from build123d import *

# Parameters (mm, degrees)
REFERENCE_R         = 6.35
REFERENCE_R_2       = 3.175
REFERENCE_R_3       = 2.0955
REFERENCE_R_4       = 1.9685
REFERENCE_R_5       = 2.032
BOSS_EXTRUDE3_DEPTH = 6.604


with BuildPart() as part:
    # reference → Boss-Extrude3 (new body)
    with BuildSketch(Plane.XY):
        Polygon((209.55, 0), (-209.55, 0), (-209.55, 170.18), (-74.93, 304.8), (74.93, 304.8), (209.55, 170.18), align=None)
        with Locations(Location((-102.87, 111.76, 0), (0, 0, 180))):
            Circle(REFERENCE_R, mode=Mode.SUBTRACT)
        with Locations(Location((102.87, 111.76, 0), (0, 0, 180))):
            Circle(REFERENCE_R, mode=Mode.SUBTRACT)
        with Locations(Location((-59.69, 254, 0), (0, 0, 180))):
            Circle(REFERENCE_R_2, mode=Mode.SUBTRACT)
        with Locations(Location((59.69, 254, 0), (0, 0, 180))):
            Circle(REFERENCE_R_2, mode=Mode.SUBTRACT)
        with Locations(Location((170.18, 25.4, 0), (0, 0, 180))):
            Circle(REFERENCE_R_3, mode=Mode.SUBTRACT)
        with Locations(Location((-170.18, 25.4, 0), (0, 0, 180))):
            Circle(REFERENCE_R_3, mode=Mode.SUBTRACT)
        with Locations(Location((83.82, 229.87, 0), (0, 0, 180))):
            Circle(REFERENCE_R_4, mode=Mode.SUBTRACT)
        with Locations(Location((35.56, 229.87, 0), (0, 0, 180))):
            Circle(REFERENCE_R_4, mode=Mode.SUBTRACT)
        with Locations(Location((83.82, 278.13, 0), (0, 0, 180))):
            Circle(REFERENCE_R_4, mode=Mode.SUBTRACT)
        with Locations(Location((35.56, 278.13, 0), (0, 0, 180))):
            Circle(REFERENCE_R_4, mode=Mode.SUBTRACT)
        with Locations(Location((24.4475, 284.48, 0), (0, 0, 180))):
            Circle(REFERENCE_R_5, mode=Mode.SUBTRACT)
        with Locations(Location((24.4475, 254.381, 0), (0, 0, 180))):
            Circle(REFERENCE_R_5, mode=Mode.SUBTRACT)
        with Locations(Location((-24.4475, 254.381, 0), (0, 0, 180))):
            Circle(REFERENCE_R_5, mode=Mode.SUBTRACT)
        with Locations(Location((-24.4475, 284.48, 0), (0, 0, 180))):
            Circle(REFERENCE_R_5, mode=Mode.SUBTRACT)
    extrude(amount=BOSS_EXTRUDE3_DEPTH)


solid = part.part
Build history of the part. All positions in model axes, mm. Round coordinates to 2 decimals unless told otherwise and drop trailing zeros. Write each loop counter-clockwise with the first axis right and the second up, starting at its lowest first coordinate (ties: lowest second). Pieces come first, ordered by that corner, then holes. Notation, with made-up numbers: M -8.75,1 L 47.25,1 A10 ccw 47.25,12 Z; hole C -2.5,23.5 d2. An arc over 180 degrees is marked long. Answer as a JSON object with one key per item and string values. Group by question number.
(1) Flat gauge pins, fed straight in: pin 1 (3 mm diameter, centred on x = 35.56, y = 278.13, fed in from -Z); pin 2 (1 mm diameter, centred on y = 246, z = 2, fed in from +X). Where does each tip first touch, or does it go through?
(2) Cut at C-C (y = 264). Give the cut face in (x, z), and give its area (3 significant figures).
(3) Drill centre lines: L1, parallel to X at y = 284.48, z = 4.75; L2, parallel to Y at x = 59.69, z = 3 (3 decimals); L3, parallel to Y at x = -99, z = 2. Where is each one in solid material? Low to high.
(4) Mould opens along Y. For faces 1 (the cylindrical face through (-101.49, 117.96, 3.26)), 2 (the flat face through (141.3, 238.43, 3.26)), 3 (the flat face through (3, 121, 6.604)) say: pulls with the +Y half, pulls with the -Y half, needs draft (parallel to the pull), parting line crosses it, or undercut.
(5) Cut at A-A (x = -102.87). Give the cut face in (y, z).
(6) Cut at D-D (x = -155). Give the cut face in (y, z), and give its area (3 significant figures).
(7) Cut at B-B (z = 4.5). Give the number of separate pieces and of enclosed holes in the cut face, and give its area (3 significant figures).
Responses:
{
 "1": {"pin 1": "passes through", "pin 2": "stops at x = 134.23"},
 "2": {"outline": "M -115.73,0 L 115.73,0 L 115.73,6.6 L -115.73,6.6 Z", "area": "1,530 mm2"},
 "3": {"L1": "x = -95.25 to -26.48, -22.42 to 22.42, 26.48 to 95.25", "L2": "y = 0 to 250.825, 257.175 to 304.8", "L3": "y = 0 to 106.73, 116.79 to 280.73"},
 "4": {"face 1": "undercut", "face 2": "pulls with the +Y half", "face 3": "needs draft"},
 "5": {"outline": "M 0,0 L 105.41,0 L 105.41,6.6 L 0,6.6 Z; M 118.11,0 L 276.86,0 L 276.86,6.6 L 118.11,6.6 Z"},
 "6": {"outline": "M 0,0 L 224.73,0 L 224.73,6.6 L 0,6.6 Z", "area": "1,480 mm2"},
 "7": {"separate pieces": "1", "enclosed holes": "14", "area": "109,000 mm2"}
}
